Here's the drawing with two shaded views (mm, measured from the low corner). I have some questions. Give positions to 0.01 mm unless a question says otherwise; leave off trailing zeros. Loops run counter-clockwise (first coordinate to the right, second up) from the corner with the lowest first, then second, coordinate; pieces in that order, holes last.
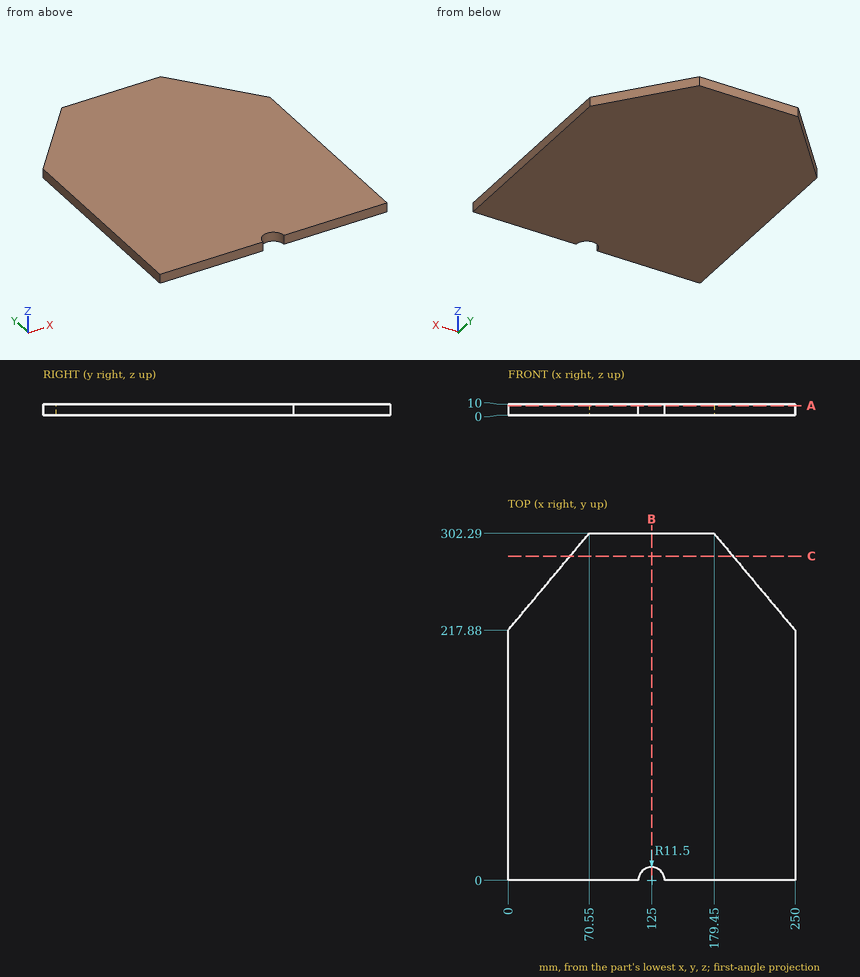
(1) Suppose I cut it at C-C on y = 282.5. List the corners of the cut face in (x, z) for me.
Returned:
outline: (54.01, 0) - (195.99, 0) - (195.99, 10) - (54.01, 10) - close
(2) Suppose I cut it at B-B on x = 125. List the corners of the cut face in (y, z) for me, plus the area to 3 significant figures.
Returned:
outline: (11.5, 0) - (302.29, 0) - (302.29, 10) - (11.5, 10) - close
area: 2,910 mm2
(3) Suppose I cut it at A-A on z = 8.5. List the corners of the cut face in (x, y) for me, plus the area to 3 significant figures.
Returned:
outline: (0, 0) - (113.5, 0) arc R11.5 cw to (136.5, 0) - (250, 0) - (250, 217.88) - (179.45, 302.29) - (70.55, 302.29) - (0, 217.88) - close
area: 69,400 mm2
(4) Will these pins go through, and if not, where does the flat tip stop? P1, Ø3, axis at y = 236, z = 8.5, coming from the -X side; P2, Ø6, axis at x = 171.5, y = 249, coming from the -Z side; P3, Ø4, axis at y = 241, z = 7, coming from the +X side.
Returned:
P1: stops at x = 13.89
P2: stops at z = 0
P3: stops at x = 232.35
(5) Please list where these lines run through material, in increasing order: probe 1 along Y at (x, z) = (201, 7.5); probe 2 along Y at (x, z) = (47, 5); probe 3 along X at (y, z) = (290, 4.5).
Returned:
probe 1: y = 0 to 276.51
probe 2: y = 0 to 274.11
probe 3: x = 60.28 to 189.72
